The listing builds one solid part. Answer for the finished solid, in the listing's coordinates (mm). Coordinates: 2 decimals unless noted, no trailing zeros. Order: outer loops, then holes, each group sorted by start corner. A loop starts at its lowest first (then second) coordinate and runs counter-clockwise, first axis right, second up. Notation, with made-up numbers: (25, -37.5) - (62, -37.5) arc R22 cw to (62, -26.5) - close; hole circle Ø7 at (10.5, 7.25). An arc over 180 degrees is marked (long way). Use a Markdown table: item, result. Add a question column.
Item 1: The part is cut by section A-A, the plane y = 11.5. Give the vertices of the cut face in (x, z) (3 decimals).
Item 2: Find the intervals of material crossed by line 1 along X through (y, z) = (68, -0.25); line 2 along Y through (x, z) = (1, 0); line 3 along Y through (x, z) = (-2, -1), in increasing order.
Item 3: The mould has two halves that part along Y. Classify faces 1 (the cylindrical face through (-1.93, 50.15, -2.52)), 2 (the conical face through (0.4, 1.19, -1.26)), 3 (the conical face through (0.4, 100.41, -1.26)): released by +Y, released by -Y, zero draft, split by the parting line, or undercut.
Item 4: Flat-ended cylindrical pins translate along their axes: P1, Ø1, axis at y = 35, z = -1.5, coming from the +X side; P2, Ø2, axis at y = 26, z = -1.5, coming from the -X side; P3, Ø3, axis at x = -0.5, z = -1.5, coming from the -Y side; P4, Ø1, axis at y = 12, z = -2, coming from the +X side. Find the tip coordinate at first contact, or state that the pin passes through.
from build123d import *

# Parameters (mm, degrees)
SKETCH1_R           = 3.175
BOSS_EXTRUDE1_DEPTH = 101.6


with BuildPart() as part:
    # Sketch1 → Boss-Extrude1 (new body)
    with BuildSketch(Plane(origin=(0, 0, 0), x_dir=(1, 0, 0), z_dir=(0, 1, 0))):
        with Locations(Location((0, 0, 0), (0, 0, 270))):
            Circle(SKETCH1_R)
    extrude(amount=BOSS_EXTRUDE1_DEPTH)

    # Sketch3 → Cut-Revolve2 (revolve, cut)
    with BuildSketch(Plane.XY, mode=Mode.PRIVATE) as cut_revolve2_sk:
        Polygon((3.175, 97.200590949), (0.635, 101.6), (3.175, 101.6), align=None)
    cut_revolve2 = revolve(cut_revolve2_sk.sketch.rotate(Axis((0, 101.6, 0), (0, -1, 0)), 270), axis=Axis((0, 101.6, 0), (0, -1, 0)), mode=Mode.SUBTRACT)

    # Mirror1: Cut-Revolve2 across plane
    add(cut_revolve2.mirror(Plane.ZX.offset(50.8)), mode=Mode.SUBTRACT)


solid = part.part
Solution:
| question | item | result |
|---|---|---|
| 1 | outline | circle Ø6.35 at (0, 0) |
| 2 | line 1 | x = -3.17 to 3.17 |
| 2 | line 2 | y = 0.63 to 100.97 |
| 2 | line 3 | y = 2.77 to 98.83 |
| 3 | face 1 | zero draft |
| 3 | face 2 | released by -Y |
| 3 | face 3 | released by +Y |
| 4 | P1 | stops at x = 3.01 |
| 4 | P2 | stops at x = -3.14 |
| 4 | P3 | stops at y = 0 |
| 4 | P4 | stops at x = 2.8 |
